```python
from build123d import *

# Parameters (mm, degrees)
F0_W     = 152.678899467
F0_H     = 151.7591327429
F1_DEPTH = 25.4
F2_DEPTH = 25.4
F3_T     = -2.54
F4_W     = 143.7006218052
F4_H     = 0.7638186216
F5_DEPTH = 25.4


with BuildPart() as f1:
    # F0 (on Top) → F1 (new body)
    with BuildSketch(Plane.XY):
        with Locations((-0.2116523683, 0.7638186216)):
            Rectangle(F0_W, F0_H)
    extrude(amount=F1_DEPTH)

    # F2 (add): a face of the model
    f2_faces = [f1.faces().sort_by_distance(p)[0] for p in [
        (-0.2116523683, 0.7638186216, 25.4),
    ]]
    extrude(f2_faces, amount=F2_DEPTH)

    # F3
    f3_openings = [f1.faces().sort_by_distance(p)[0] for p in [
        (-0.211652, 0.763819, 50.8),
    ]]
    offset(amount=F3_T, openings=f3_openings)

    # F4 (on face) → F5 (join)
    with BuildSketch(Plane.XY.offset(2.54)):
        with Locations((-2.1607911992, 0.3819093108)):
            Rectangle(F4_W, F4_H)
    extrude(amount=F5_DEPTH)


solid = f1.part
```
Model file for the job. Use its own axes, mm. A direction names the side the tool comes from. Give positions to 0.01 mm unless a question says otherwise; leave off trailing zeros. Order: outer loops, then holes, each group sorted by start corner. A loop starts at its lowest first (then second) coordinate and runs counter-clockwise, first axis right, second up.
1) Mould opens along X. For faces 1 (the flat face through (-1, 76.643, 25)), 2 (the flat face through (-76.551, 0, 25)), 3 (the flat face through (-74.011, -0.3, 26.3)) say: +X half, -X half, draft (parallel to the pull), parting line (faces both ways), or undercut.
2) Wall check: probe 1 along Y at (x, z) = (-32.5, 5); probe 2 along X at (y, z) = (-10, 14); probe 3 along Y at (x, z) = (-6.5, 46). Give the ranges that are in metal, low to high.
3) Pin check, flat tips, straight feed: pin 1 (0.6 mm diameter, centred on x = 30, y = 0.5, fed in from +Z); pin 2 (3 mm diameter, centred on x = 26, y = 33, fed in from +Z); pin 3 (8 mm diameter, centred on x = 50.5, y = -57, fed in from -Z). Stop position of each tip, or through.
4) Saw through at D-D, the plane z = 47. Write the cut outline in (x, y), then the cut area to 3 significant figures.
5) Saw through at A-A, the plane z = 11. Write the cut outline in (x, y).
6) Saw through at C-C, the plane x = -13. Write the cut outline in (y, z), then the cut area to 3 significant figures.
7) 3-axis set-ups, long thin cutter, end or side, ignore diameter. For faces 4 (the flat face through (-1, -75.116, 25)), 5 (the flat face through (-3, 0, 15)): which of +Z, -Z, +X, -X, +Y, -Y reach the whole face in a straight line?
8) Saw through at B-B, the plane y = 49.5. Write the cut outline in (x, z).
Computed:
1. face 1: draft
1. face 2: -X half
1. face 3: undercut
2. probe 1: y = -75.12 to -72.58, 0 to 0.76, 74.1 to 76.64
2. probe 2: x = -76.55 to -74.01, 73.59 to 76.13
2. probe 3: y = -75.12 to -72.58, 74.1 to 76.64
3. pin 1: stops at z = 27.94
3. pin 2: stops at z = 2.54
3. pin 3: stops at z = 0
4. outline: (-76.55, -75.12) - (76.13, -75.12) - (76.13, 76.64) - (-76.55, 76.64) - close; hole (-74.01, -72.58) - (73.59, -72.58) - (73.59, 74.1) - (-74.01, 74.1) - close
4. area: 1,520 mm2
5. outline: (-76.55, -75.12) - (76.13, -75.12) - (76.13, 76.64) - (-76.55, 76.64) - close; hole (-74.01, -72.58) - (73.59, -72.58) - (73.59, 74.1) - (-74.01, 74.1) - (-74.01, 0.76) - (69.69, 0.76) - (69.69, 0) - (-74.01, 0) - close
6. outline: (-75.12, 0) - (76.64, 0) - (76.64, 50.8) - (74.1, 50.8) - (74.1, 2.54) - (0.76, 2.54) - (0.76, 27.94) - (0, 27.94) - (0, 2.54) - (-72.58, 2.54) - (-72.58, 50.8) - (-75.12, 50.8) - close
6. area: 650 mm2
7. face 4: +Z, -Z, +X, -X, -Y
7. face 5: +Z
8. outline: (-76.55, 0) - (76.13, 0) - (76.13, 50.8) - (73.59, 50.8) - (73.59, 2.54) - (-74.01, 2.54) - (-74.01, 50.8) - (-76.55, 50.8) - close
